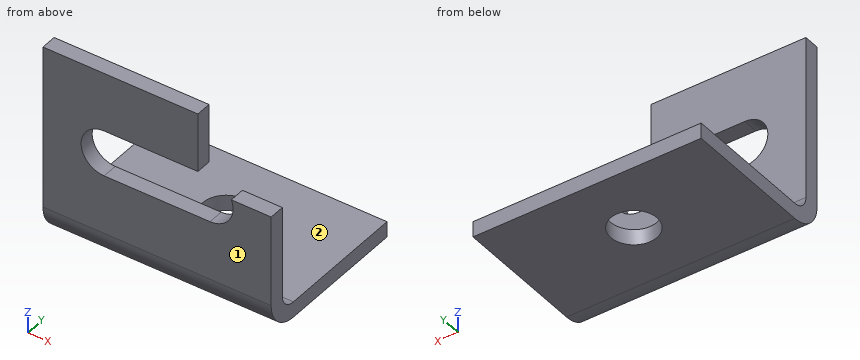
Autodesk Inventor part; units mm, degrees
ref_plane "YZ Plane" through (0, 0, 0) normal (1, 0, 0) x (0, 1, 0)
ref_plane "XZ Plane" through (0, 0, 0) normal (0, 1, 0) x (-1, 0, 0)
ref_plane "XY Plane" through (0, 0, 0) normal (0, 0, 1) x (1, 0, 0)
sketch "Sketch1" plane through (0, 0, 0) normal (0, 1, 0) x (-1, 0, 0)
  line L0 (11.1125, 9.525) -> (-11.1125, 9.525)
  line L1 (-11.1125, 9.525) -> (-11.1125, -9.525)
  line L2 (-11.1125, -9.525) -> (11.1125, -9.525)
  line L3 (11.1125, -9.525) -> (11.1125, 9.525)
  line L4 (11.1125, 9.525) -> (-11.1125, -9.525) construction
  line L5 (-11.1125, 9.525) -> (11.1125, -9.525) construction
  point P0 (0, 0)
  dimension "d0" = 22.225
  dimension "d1" = 19.05
extrude "Plate1" add sketch "Sketch1" along normal blind 1.524
sketch "Sketch2" plane through (-11.1125, 0, -8.001) normal (0, 0, -1) x (-1, 0, 0)
  line L0 (-22.225, 0) -> (0, 0)
  line L1 (0, 0) -> (0, 15.875)
  line L2 (0, 15.875) -> (-22.225, 15.875)
  line L3 (-22.225, 15.875) -> (-22.225, 0)
edge flange "Flange1" height 15.875 angle 90 thickness 1.524 bend radius 1.524 thickness toward (0, 0, -1) relief tear relief width 1.524 relief depth 0.762 edges at (0, 1.524, -9.525) wall of the first edge with corners at (11.1125, 0, -8.001) (-11.1125, 0, -8.001) (-11.1125, 15.875, -8.001) (11.1125, 15.875, -8.001)
bend "Bend1"
corner "Corner1"
sketch "Sketch3" plane through (0, 1.524, 0) normal (0, 1, 0) x (1, 0, 0)
  line L0 (11.1125, 6.477) -> (-11.1125, 6.477)
  line L1 (-11.1125, -9.525) -> (-11.1125, 6.477)
  line L2 (11.1125, -9.525) -> (-11.1125, -9.525)
  line L3 (11.1125, 6.477) -> (11.1125, -9.525)
  line L4 (-11.1125, -1.524) -> (11.1125, -1.524) construction
  line L5 (0, 6.477) -> (0, -9.525) construction
  circle A0 centre (0, -1.524) radius 2.2479
  line L6 (-5.1562, -1.524) -> (5.1562, -1.524) construction
  line L7 (-5.1562, 0.7239) -> (5.1562, 0.7239)
  line L8 (5.1562, -3.7719) -> (-5.1562, -3.7719)
  arc A1 (-5.1562, 0.7239) -> (-5.1562, -3.7719) centre (-5.1562, -1.524) ccw
  arc A2 (5.1562, -3.7719) -> (5.1562, 0.7239) centre (5.1562, -1.524) ccw
  point P0 (0, 0)
  dimension "d13" = 16.002
  dimension "d14" = 22.225
  dimension "d24" = 4.4958
  dimension "d25" = 3.7084
sketch "Sketch4" plane through (-11.1125, 15.875, -8.001) normal (0, 0, 1) x (1, 0, 0)
  line L0 (0, -12.827) -> (22.225, -12.827)
  line L1 (22.225, 0) -> (22.225, -12.827)
  line L2 (22.225, 0) -> (0, 0)
  line L3 (0, 0) -> (0, -12.827)
  line L4 (0, -6.4135) -> (22.225, -6.4135) construction
  line L5 (22.225, 0) -> (22.225, -12.827) construction
  line L6 (11.1125, -12.827) -> (11.1125, 0) construction
  line L7 (22.225, 0) -> (0, 0) construction
  point P0 (11.1125, -15.875)
  point P1 (11.1125, -6.4135)
  dimension "d15" = 22.225
  dimension "d16" = 12.827
hole "Hole1" at (0, 9.4615, -8.001) direction (0, 0, -1) diameter 4.4958 depth 1.524 tip angle 118
extrude "Cut1" cut sketch "Sketch3" against normal blind 1.524 contours A0 | A0 L7 A2 L8 | A0 L8 A1 L7
sketch "Sketch7" plane through (11.1125, 15.875, -9.525) normal (0, 0, -1) x (-1, 0, 0)
  line L0 (0, 0) -> (22.225, 0)
  line L1 (22.225, -15.875) -> (0, -15.875)
  line L2 (0, -12.827) -> (22.225, -12.827)
  point P0 (11.1125, -15.875)
  dimension "d28" = 15.875
  dimension "d29" = 12.827
  dimension "d30" = 22.225
sketch "Sketch8" plane through (0, 0, 0) normal (0, -1, 0) x (1, 0, 0)
  arc A0 (-5.1562, 3.7719) -> (-5.1562, -0.7239) centre (-5.1562, 1.524) ccw
  line L0 (-5.1562, 3.7719) -> (5.1562, 3.7719)
  arc A1 (5.1562, -0.7239) -> (5.1562, 3.7719) centre (5.1562, 1.524) ccw
  line L1 (5.1562, -0.7239) -> (-5.1562, -0.7239)
  line L2 (-11.1125, -6.477) -> (11.1125, -6.477)
  line L3 (11.1125, 9.525) -> (11.1125, -6.477)
  line L4 (-11.1125, 9.525) -> (11.1125, 9.525)
  line L5 (-11.1125, -6.477) -> (-11.1125, 9.525)
  line L6 (11.1125, -9.525) -> (-11.1125, -9.525)
  line L7 (11.1125, -6.477) -> (11.1125, -9.525)
  line L8 (-11.1125, -6.477) -> (11.1125, -6.477)
  line L9 (-11.1125, -9.525) -> (-11.1125, -6.477)
  point P0 (0, 0)
  dimension "d31" = 19.05
  dimension "d32" = 16.002
sketch "Sketch9" plane through (0, 1.524, 0) normal (0, 1, 0) x (1, 0, 0)
  arc A0 (5.1562, -3.7719) -> (5.1562, 0.7239) centre (5.1562, -1.524) ccw
  arc A1 (-5.1562, 0.7239) -> (-5.1562, -3.7719) centre (-5.1562, -1.524) ccw
  line L0 (5.1562, -3.7719) -> (-5.1562, -3.7719)
  line L1 (-5.1562, 0.7239) -> (5.1562, 0.7239)
  circle A2 centre (0, -1.524) radius 2.2479
  point P0 (0, 0)
  dimension "d34" = 5.1562
sketch "Sketch10" plane through (-11.1125, 15.875, -9.525) normal (0, 1, 0) x (1, 0, 0)
  line L0 (22.225, -19.05) -> (0, -19.05)
  line L1 (22.225, 0) -> (0, 0)
  line L2 (0, -1.524) -> (0, 0)
  line L3 (0, -1.524) -> (0, -3.048)
  line L4 (0, -19.05) -> (0, -3.048)
  line L5 (0, 0) -> (7.1374, 0)
  line L6 (7.1374, 0) -> (7.1374, -19.05)
  line L7 (7.1374, -19.05) -> (0, -19.05)
  line L8 (0, -19.05) -> (0, 0)
  line L9 (22.225, 0) -> (15.0876, 0)
  line L10 (15.0876, 0) -> (15.0876, -19.05)
  line L11 (15.0876, -19.05) -> (22.225, -19.05)
  line L12 (22.225, -19.05) -> (22.225, 0)
  line L13 (22.225, -3.048) -> (22.225, -19.05)
  line L14 (0, -19.05) -> (22.225, -19.05)
  line L15 (22.225, -19.05) -> (22.225, -11.9126)
  line L16 (22.225, -11.9126) -> (0, -11.9126)
  line L17 (0, -11.9126) -> (0, -19.05)
  line L18 (0, -19.05) -> (7.1374, -19.05)
  line L19 (7.1374, -19.05) -> (7.1374, -11.9126)
  line L20 (7.1374, -11.9126) -> (0, -11.9126)
  line L21 (0, -11.9126) -> (0, -19.05)
  line L22 (22.225, -19.05) -> (15.0876, -19.05)
  line L23 (15.0876, -19.05) -> (15.0876, -11.9126)
  line L24 (15.0876, -11.9126) -> (22.225, -11.9126)
  line L25 (22.225, -11.9126) -> (22.225, -19.05)
  point P0 (11.1125, -9.525)
  dimension "d35" = 7.1374
  dimension "d36" = 7.1374
  dimension "d37" = 7.1374
extrude "Cut2" cut sketch "Sketch10" against normal through all contours L0 L10 L16 L12
equation "\"d22\" = Thickness"
equation "\"d26\" = Thickness"
equation "\"d36\" = d35"
equation "\"d38\" = Thickness"
equation "\"d3\" = BendReliefWidth"
equation "\"d4\" = BendReliefDepth"
equation "\"d5\" = MinimumRemnant"
equation "\"d6\" = BendRadius"
equation "\"d9\" = BendRadius"
equation "\"d10\" = CornerReliefSize"
equation "\"d11\" = GapSize"
equation "\"d12\" = JacobiRadiusSize"
equation "\"BendRadius\" = Thickness"
equation "\"BendReliefWidth\" = Thickness"
equation "\"BendReliefDepth\" = 0.5 * Thickness"
equation "\"CornerReliefSize\" = 4 * Thickness"
equation "\"MinimumRemnant\" = 2 * Thickness"
equation "\"TransitionRadius\" = BendRadius"
equation "\"JacobiRadiusSize\" = BendRadius"
equation "\"GapSize\" = Thickness"
equation "\"d2\" = BendRadius"
properties part number "Bracket (15275A53)_RightCut" material "Steel"
Can you work these out from the model? Positions are in its coordinate system, mm. Face numbers are marked on the shaded views. A direction names the side the tool comes from. Give positions to 0.01 mm unless a question says otherwise; leave off trailing zeros. Loops run counter-clockwise (first coordinate to the right, second up) from the corner with the lowest first, then second, coordinate; pieces in that order, holes last. Notation, with made-up numbers: M -25.5,-26.5 L 16.5,-26.5 A18 cw 16.5,-18.5 Z; hole C 4.5,87 d9. An arc over 180 degrees is marked long. Use CSV: the item, a comma, the result in double quotes. Start each with the question number.
1. Imagine slicing it at C-C, the plane x = 3. Write out the boundary of the cut face in (y, z) (3 decimals), plus the area to 3 significant figures.
2. Imagine slicing it at B-B, the plane z = 1.5. Write out the boundary of the cut face in (x, y), plus the area to 3 significant figures.
3. Imagine slicing it at D-D, the plane z = 5.25. Write out the boundary of the cut face in (x, y).
4. On a 3-axis mill with a long thin cutter (end or side, diameter ignored), from which of +Z, -Z, +X, -X, +Y, -Y can I reach the whole of each face in a straight line? I mean the marked faces 1 and 2. Say none if no direction works.
5. For P1, Ø0.8, axis at x = 10, y = 1, coming from the +Z side; P2, Ø8, axis at x = -9, y = 9.5, coming from the +Z side; P3, Ø0.5, axis at y = 1, z = 6, coming from the +X side, each with a flat end and sliding along its axis, tell me the tip position at first contact or that it passes through.
6. Imagine slicing it at A-A, the plane x = 0. Write out the boundary of the cut face in (y, z) (3 decimals), plus the area to 3 significant figures.
7. If I drill on L1, parallel to Z at x = -2, y = 5.5 (3 decimals); L2, parallel to Y at x = 0, z = -8.8 (3 decimals); L3, parallel to Y at x = -1.75, z = 8.5, over which ranges is the centre line in solid material (lowest first)?
Response values:
1,outline,"M 0,-6.477 A3.048 ccw 3.048,-9.525 L 15.875,-9.525 L 15.875,-8.001 L 3.048,-8.001 A1.524 cw 1.524,-6.477 L 1.524,-0.724 L 0,-0.724 Z; M 0,3.772 L 1.524,3.772 L 1.524,9.525 L 0,9.525 Z"
1,area,"42.6 mm^2"
2,outline,"M -11.11,0 L -7.4,0 L -7.4,1.52 L -11.11,1.52 Z; M 7.4,0 L 11.11,0 L 11.11,1.52 L 7.4,1.52 Z"
2,area,"11.3 mm^2"
3,outline,"M -11.11,0 L 3.98,0 L 3.98,1.52 L -11.11,1.52 Z"
4,face 1,"+Z, -Z, +X, -X, -Y"
4,face 2,"+Z, +X, -X, +Y"
5,P1,"z = 2.39"
5,P2,"z = -8"
5,P3,"x = 3.98"
6,outline,"M 0,-6.477 A3.048 ccw 3.048,-9.525 L 7.214,-9.525 L 7.214,-8.001 L 3.048,-8.001 A1.524 cw 1.524,-6.477 L 1.524,-0.724 L 0,-0.724 Z; M 0,3.772 L 1.524,3.772 L 1.524,9.525 L 0,9.525 Z; M 11.709,-9.525 L 15.875,-9.525 L 15.875,-8.001 L 11.709,-8.001 Z"
6,area,"35.7 mm^2"
7,L1,"-9.525 to -8.001"
7,L2,"1.075 to 7.214, 11.709 to 15.875"
7,L3,"0 to 1.52"
